The figure shows three views and two pictorial views of one solid part (mm, origin at its lowest corner). Answer the questions. Coordinates: 2 decimals unless noted, no trailing zeros. Order: outer loops, then holes, each group sorted by start corner. A loop starts at its lowest first (then second) coordinate and runs counter-clockwise, first axis right, second up. Notation, with made-up numbers: (22, -0.5) -> (38, -0.5) arc R21 cw to (38, 22.5) -> close; hole circle Ø9 at (83, 12). An arc over 180 degrees is marked (long way). Use one line per item in the form item = value.
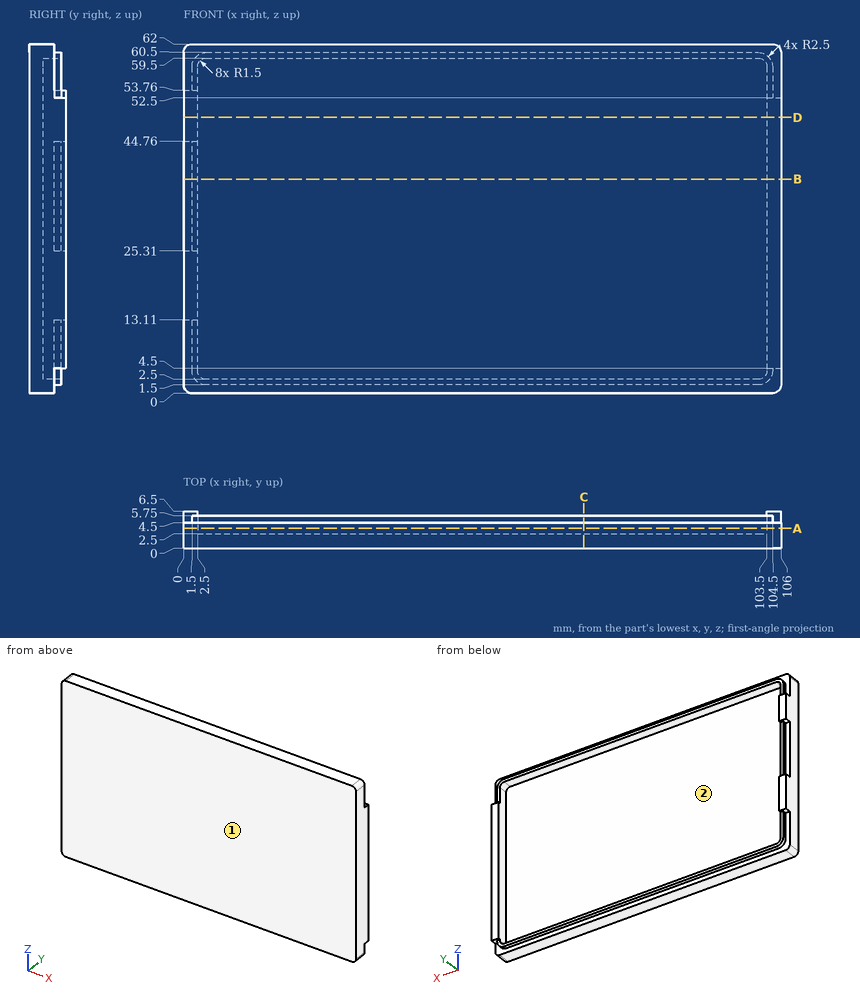
(1) Straight lines are drawn through the part: line 1 along Z through (x, y) = (77, 3.5); line 2 along X through (y, z) = (6, 23.5); line 3 along X through (y, z) = (5.5, 35.5). For each, find the intervals that lie inside material, in ascending order.
Data:
line_1 = 0 to 2.5, 59.5 to 62
line_2 = 0 to 2.5, 103.5 to 106
line_3 = 1.5 to 2.5, 103.5 to 106
(2) The mould has two halves that part along X. Classify the marked faces 1 and 2: released by +X, released by -X, zero draft, split by the parting line, or undercut.
Data:
face_1 = zero draft
face_2 = undercut
(3) Section C-C on x = 71 is taken. Write down the section's boundary in (y, z).
Data:
outline = (0, 0) -> (4.5, 0) -> (4.5, 1.5) -> (5.75, 1.5) -> (5.75, 2.5) -> (2.5, 2.5) -> (2.5, 59.5) -> (5.75, 59.5) -> (5.75, 60.5) -> (4.5, 60.5) -> (4.5, 62) -> (0, 62) -> close
(4) Section B-B on z = 38 is taken. Write down the section's boundary in (x, y), plus the area to 3 significant figures.
Data:
outline = (0, 0) -> (106, 0) -> (106, 6.5) -> (103.5, 6.5) -> (103.5, 2.5) -> (2.5, 2.5) -> (2.5, 5.75) -> (1.5, 5.75) -> (1.5, 4.5) -> (0, 4.5) -> close
area = 281 mm²
(5) Each of these flat-tipped pins is pushed along its axis until it touches: P1, Ø1, axis at y = 5.5, z = 56.5, coming from the +X side; P2, Ø1.6, axis at x = 1.5, y = 5.5, coming from the -Z side; P3, Ø6, axis at x = 74.5, z = 4.5, coming from the +Y side. Where does it stop, or does it pass through?
Data:
P1 = 104.5
P2 = 2.17
P3 = 5.75
(6) Section D-D on z = 49 is taken. Write down the section's boundary in (x, y).
Data:
outline = (0, 0) -> (106, 0) -> (106, 6.5) -> (103.5, 6.5) -> (103.5, 2.5) -> (2.5, 2.5) -> (2.5, 6.5) -> (0, 6.5) -> close
(7) Section A-A on y = 3.5 is taken. Write down the section's boundary in (x, z).
Data:
outline = (0, 1.5) arc R1.5 ccw to (1.5, 0) -> (104.5, 0) arc R1.5 ccw to (106, 1.5) -> (106, 60.5) arc R1.5 ccw to (104.5, 62) -> (1.5, 62) arc R1.5 ccw to (0, 60.5) -> close; hole (2.5, 4) arc R1.5 ccw to (4, 2.5) -> (102, 2.5) arc R1.5 ccw to (103.5, 4) -> (103.5, 58) arc R1.5 ccw to (102, 59.5) -> (4, 59.5) arc R1.5 ccw to (2.5, 58) -> close
